Geometry: see drawing. Coordinates: mm, zero at the bounding-box minimum. Coordinates: 2 decimals unless noted, no trailing zeros. Write each loop counter-clockwise with the first axis right and the second up, starting at its lowest first coordinate (ties: lowest second). Pieces come first, ordered by that corner, then holes. Notation, with made-up numbers: (15, 53.25) -> (40, 53.25) arc R8 ccw to (40, 62.25) -> close; hole circle Ø2 at (21.25, 18). An arc over 180 degrees is marked (long way). Use one line per item in the form item = value. Start each with the question number.
(1) Pull-direction query (Z, two-part tool) for the marked faces 1, 2, 3 and 4; classes: released by +Z, released by -Z, zero draft, split by the parting line, or undercut.
(2) Cut plane A-A on x = 46. Return the cut outline in (y, z) (3 decimals).
(3) Cut plane B-B on y = 10.5. Return the cut outline in (x, z), plus the area to 3 significant figures.
(4) Ray query, line 1 along Z through (x, y) = (28.5, 4); line 2 along Y through (x, z) = (46, 1) (3 decimals); line 3 along Z through (x, y) = (11.5, 20). Return the intervals inside material, ascending.
(5) Cut plane C-C on z = 2.25. Return the cut outline in (x, y) (3 decimals).
(6) First-contact query: pin 1 (3.5 mm diameter, centred on x = 4, y = 29.625, fed in from +Z); pin 2 (1.5 mm diameter, centred on x = 22, y = 19.5, fed in from +Z); pin 3 (0.9 mm diameter, centred on x = 36, z = 5, fed in from +Y). Flat tips, straight axial feed; report the tip coordinate or a pass-through.
(7) Cut plane D-D on x = 40. Return the cut outline in (y, z).
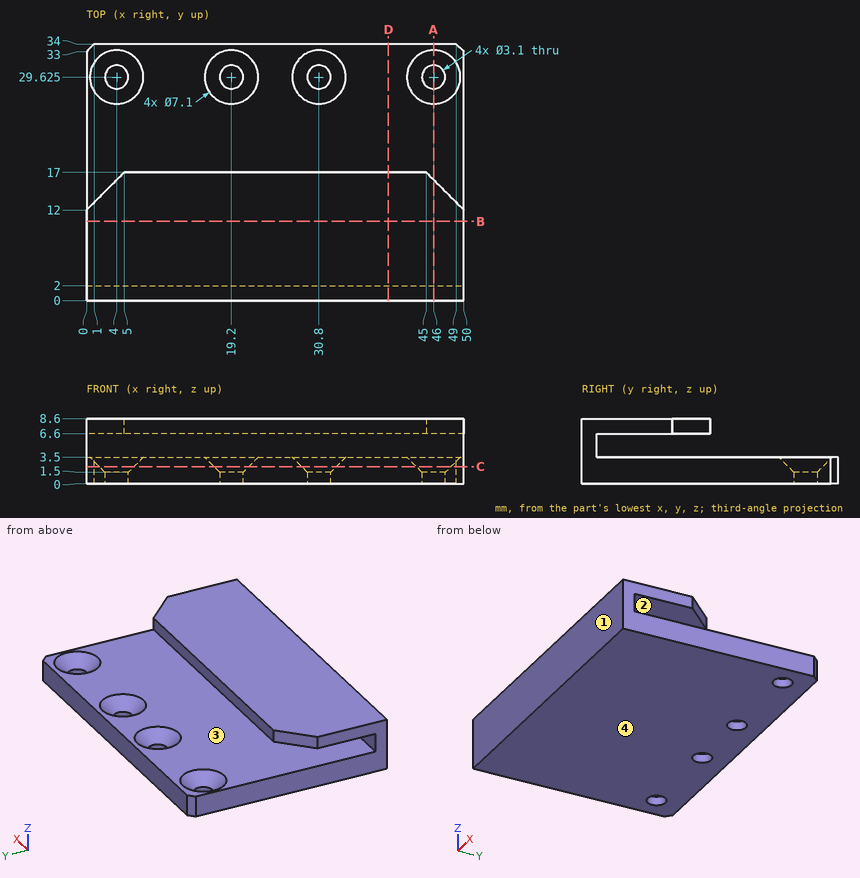
Values:
q1.face_1 = zero draft
q1.face_2 = undercut
q1.face_3 = undercut
q1.face_4 = released by -Z
q2.outline = (0, 0) -> (28.075, 0) -> (28.075, 1.5) -> (26.075, 3.5) -> (2, 3.5) -> (2, 6.6) -> (16, 6.6) -> (16, 8.6) -> (0, 8.6) -> close; (31.175, 0) -> (34, 0) -> (34, 3.5) -> (33.175, 3.5) -> (31.175, 1.5) -> close
q3.outline = (0, 0) -> (50, 0) -> (50, 3.5) -> (0, 3.5) -> close; (0, 6.6) -> (50, 6.6) -> (50, 8.6) -> (0, 8.6) -> close
q3.area = 275 mm2
q4.line_1 = 0 to 3.5, 6.6 to 8.6
q4.line_2 = 0 to 28.075, 31.175 to 34
q4.line_3 = 0 to 3.5
q5.outline = (0, 0) -> (50, 0) -> (50, 33) -> (49, 34) -> (1, 34) -> (0, 33) -> close; hole circle Ø4.6 at (4, 29.625); hole circle Ø4.6 at (19.2, 29.625); hole circle Ø4.6 at (30.8, 29.625); hole circle Ø4.6 at (46, 29.625)
q6.pin_1 = 1.7
q6.pin_2 = 3.5
q6.pin_3 = 2
q7.outline = (0, 0) -> (34, 0) -> (34, 3.5) -> (2, 3.5) -> (2, 6.6) -> (17, 6.6) -> (17, 8.6) -> (0, 8.6) -> close
